```python
from build123d import *

# Parameters (mm, degrees)
BOSS_EXTRUDE1_DEPTH     = 60
SKETCH2_R               = 20
BOSS_EXTRUDE2_DEPTH     = 1
SKETCH3_R               = 21
BOSS_EXTRUDE3_DEPTH     = 111.072
SKETCH4_R               = 9
BOSS_EXTRUDE4_DEPTH     = 20
CUT_EXTRUDE1_DEPTH      = 187.415206418
CUT_EXTRUDE1_DEPTH_BACK = 187.415206418
SKETCH5_R               = 3.2
BOSS_EXTRUDE5_START     = 24
SKETCH6_R               = 9
BOSS_EXTRUDE5_DEPTH     = 24
CUT_EXTRUDE2_DEPTH      = 209.657818411
CUT_EXTRUDE2_DEPTH_BACK = 209.657818411
SKETCH7_R               = 3.2
BOSS_EXTRUDE6_DEPTH     = 6


with BuildPart() as part:
    # Sketch1 → Boss-Extrude1 (new body)
    with BuildSketch(Plane(origin=(0, 0, 0), x_dir=(1, 0, 0), z_dir=(0, 1, 0))):
        with BuildLine():
            Line((21, 0), (21, -40))
            ThreePointArc((21, -40), (0, -61), (-21, -40))
            Line((-21, -40), (-21, 0))
            ThreePointArc((-21, 0), (0, 21), (21, 0))
        make_face()
    extrude(amount=BOSS_EXTRUDE1_DEPTH)

    # Sketch2 → Boss-Extrude2 (add)
    with BuildSketch(Plane(origin=(0, 60, 0), x_dir=(1, 0, 0), z_dir=(0, 1, 0))):
        with Locations(Location((0, -40, 0), (0, 0, 270))):
            Circle(SKETCH2_R)
    extrude(amount=BOSS_EXTRUDE2_DEPTH)

    # Sketch3 → Boss-Extrude3 (add)
    with BuildSketch(Plane(origin=(0, 60, 0), x_dir=(1, 0, 0), z_dir=(0, 1, 0))):
        with Locations(Location((0, 0, 0), (0, 0, 180))):
            Circle(SKETCH3_R)
    extrude(amount=BOSS_EXTRUDE3_DEPTH)

    # Sketch4 → Boss-Extrude4 (add)
    with BuildSketch(Plane.XZ):
        with Locations(Location((0, 3, 0), (0, 0, 90))):
            Circle(SKETCH4_R)
    extrude(amount=BOSS_EXTRUDE4_DEPTH)

    # Sketch5 → Cut-Extrude1 (cut, two sides: drawn at the far end of the back side and taken through both)
    with BuildSketch(Plane.ZY.offset(21).offset(-CUT_EXTRUDE1_DEPTH_BACK)):
        with Locations((3, -12)):
            Circle(SKETCH5_R)
    extrude(amount=CUT_EXTRUDE1_DEPTH + CUT_EXTRUDE1_DEPTH_BACK, mode=Mode.SUBTRACT)

    # Sketch6 → Boss-Extrude5 (add)
    with BuildSketch(Plane(origin=(0, 171.072, 0), x_dir=(1, 0, 0), z_dir=(0, 1, 0)).offset(BOSS_EXTRUDE5_START)):
        with Locations(Location((0, -3, 0), (0, 0, 270))):
            Circle(SKETCH6_R)
    extrude(amount=-BOSS_EXTRUDE5_DEPTH)

    # Sketch7 → Cut-Extrude2 (cut, two sides: drawn at the far end of the back side and taken through both)
    with BuildSketch(Plane.ZY.offset(21).offset(-CUT_EXTRUDE2_DEPTH_BACK)):
        with Locations((3, 183.072)):
            Circle(SKETCH7_R)
    extrude(amount=CUT_EXTRUDE2_DEPTH + CUT_EXTRUDE2_DEPTH_BACK, mode=Mode.SUBTRACT)

    # Sketch8 → Boss-Extrude6 (add)
    with BuildSketch(Plane.XZ):
        Polygon((19.5, 47.794228634), (36.820508076, 57.794228634), (33.820508076, 62.990381057), (16.5, 52.990381057), align=None)
    extrude(amount=-BOSS_EXTRUDE6_DEPTH)


solid = part.part
```
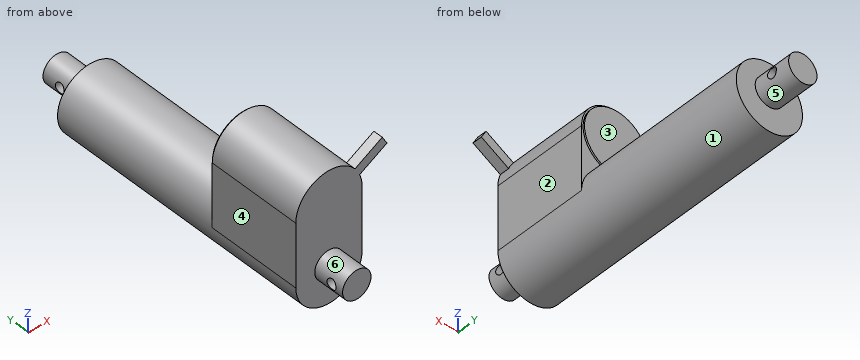
Input: part model. Units: mm. Frame: model coordinates. Face numbers are marked on the shaded views. A direction names the side the tool comes from. Give positions to 0.01 mm unless a question says otherwise; leave off trailing zeros. Write each loop counter-clockwise with the first axis right and the second up, starting at its lowest first coordinate (ties: lowest second). Pieces come first, ordered by that corner, then holes. Notation, with made-up numbers: (62.25, 86) - (73.25, 86) arc R19 cw to (73.25, 105) - close; hole circle Ø1 at (-18.5, 72.5). An arc over 180 degrees is marked (long way). Write item = value, one per line. Start each with the question number.
1. Section query D-D, the plane y = 157. Output: boundary loops of the cut face in (x, z), then the cut area to 3 significant figures.
2. Ray query, L1, parallel to Y at x = -4, z = 3; L2, parallel to Y at x = -16, z = 21.5; L3, parallel to X at y = 25, z = 16. Return the intervals inside material, ascending.
3. Section query A-A, the plane z = 3. Output: boundary loops of the cut face in (x, y), then the cut area to 3 significant figures.
4. Mould query, pull axis X, two halves, no side actions, for the marked faces 1, 2 and 3. Classes: released by +X, released by -X, zero draft, split by the parting line, or undercut.
5. Section query C-C, the plane z = 16.5. Output: boundary loops of the cut face in (x, y), then the cut area to 3 significant figures.
6. Access query for the marked faces 4, 5 and 6. Directions: +Z, -Z, +X, -X, +Y, -Y. A direction counts if a zero-diameter tool reaches every point of the face in a straight line with its end or side. Return the directions, or none.
7. First-contact query: pin 1 Ø2 at (x, y) = (6.5, 7) entering from +Z; pin 2 Ø10 at (y, z) = (-12, 3) entering from +X; pin 3 Ø12.5 at (x, z) = (-1.5, 34.5) entering from +Y. Flat tips, straight axial feed; report the tip coordinate or a pass-through.
8. Section query B-B, the plane x = 0. Output: boundary loops of the cut face in (y, z), then the cut area to 3 significant figures.
Check sheet entries:
q1.outline = circle Ø42 at (0, 0)
q1.area = 1,390 mm2
q2.L1 = -20 to -15.2, -8.8 to 179.87, 186.27 to 195.07
q2.L2 = 0 to 60
q2.L3 = -21 to 21
q3.outline = (-21, 0) - (-9, 0) - (-9, -8.8) - (9, -8.8) - (9, 0) - (21, 0) - (21, 60) - (20.78, 60) - (20.78, 171.07) - (9, 171.07) - (9, 179.87) - (-9, 179.87) - (-9, 171.07) - (-20.78, 171.07) - (-20.78, 60) - (-21, 60) - close; (-9, -20) - (9, -20) - (9, -15.2) - (-9, -15.2) - close; (-9, 186.27) - (9, 186.27) - (9, 195.07) - (-9, 195.07) - close
q3.area = 7,700 mm2
q4.face_1 = split by the parting line
q4.face_2 = released by +X
q4.face_3 = zero draft
q5.outline = (-21, 0) - (21, 0) - (21, 60) - (12.99, 60) - (12.99, 171.07) - (-12.99, 171.07) - (-12.99, 60) - (-21, 60) - close
q5.area = 5,410 mm2
q6.face_4 = +Z, -Z, -X, +Y, -Y
q6.face_5 = +Y
q6.face_6 = -Y
q7.pin_1 = 60.27
q7.pin_2 = 9
q7.pin_3 = 61
q8.outline = (-20, -6) - (0, -6) - (0, -21) - (171.07, -21) - (171.07, -6) - (195.07, -6) - (195.07, 12) - (171.07, 12) - (171.07, 21) - (61, 21) - (61, 60) - (60, 60) - (60, 61) - (0, 61) - (0, 12) - (-20, 12) - close; hole circle Ø6.4 at (-12, 3); hole circle Ø6.4 at (183.07, 3)
q8.area = 10,400 mm2
